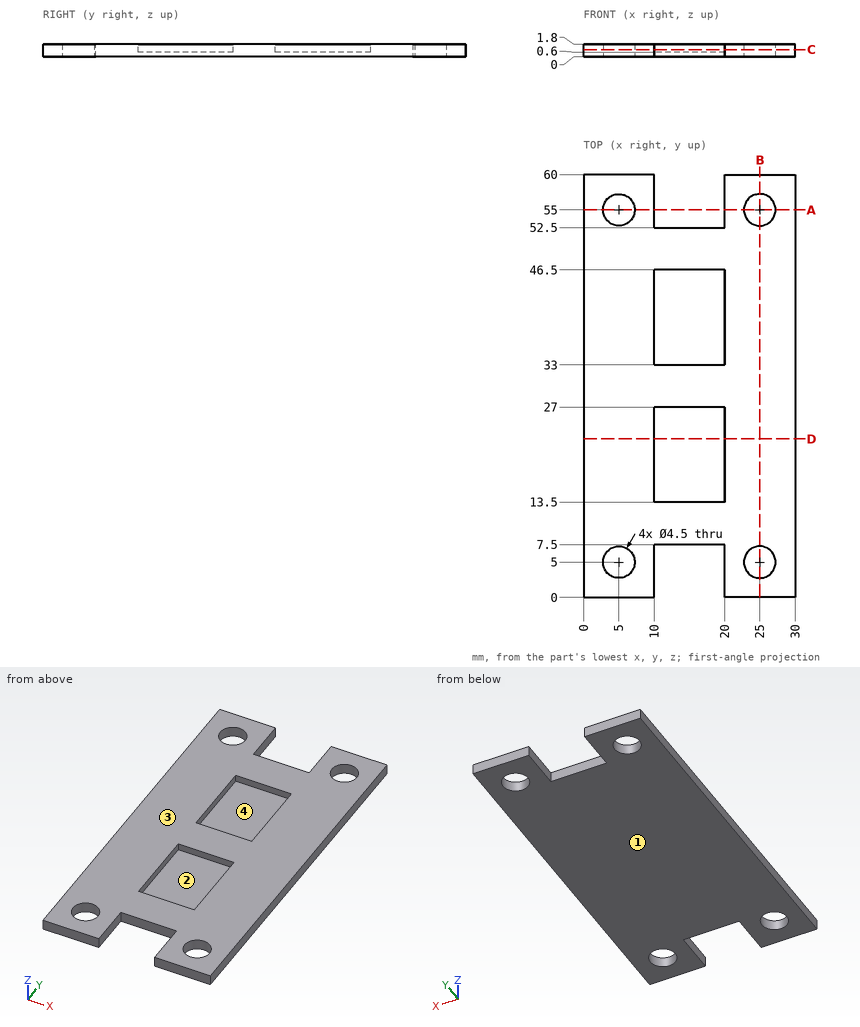
Geometry check sheet. Reference: drawing and pictorial views, mm from the part's lowest x, y, z. A direction names the side the tool comes from. Coordinates: 2 decimals unless noted, no trailing zeros. Order: outer loops, then holes, each group sorted by start corner. A loop starts at its lowest first (then second) coordinate and runs counter-clockwise, first axis right, second up. Notation, with made-up numbers: M 68,29 L 81,29 A28 cw 81,68 Z; hole C -30.75,46.5 d3. An arc over 180 degrees is marked long. Write each question's results on one line, items separated by ' | '. Start each with the question number.
1. Access from +Z, -Z, +X, -X, +Y, -Y to the whole of each face (thin tool, end or side, straight path). Record for the marked faces 3 and 4.
2. Material ranges on probe 1 along Y at (x, z) = (5, 1.4); probe 2 along Y at (x, z) = (17, 1); probe 3 along X at (y, z) = (14, 1.6), recorded low to high.
3. Go/stop test with flat-tipped pins: P1, Ø0.6, axis at y = 17, z = 1.5, coming from the -X side; P2, Ø1, axis at x = 15.5, z = 1, coming from the +Y side; P3, Ø0.5, axis at x = 13, z = 1, coming from the -Y side; P4, Ø3.5, axis at x = 25, y = 5, coming from the +Z side. Record where each tip stops, or that it passes through.
4. Mould release check, pull along X, two halves, no side actions. Record for the marked faces 1 and 2: +X half, -X half, draft (parallel to the pull), parting line (faces both ways), or undercut.
5. Cross-section at C-C on z = 1. Record the cut outline in (x, y).
6. Cross-section at D-D on y = 22.5. Record the cut outline in (x, z), and give its area (3 significant figures).
7. Cross-section at B-B on x = 25. Record the cut outline in (y, z).
8. Cross-section at A-A on y = 55. Record the cut outline in (x, z), and give its area (3 significant figures).
Checks:
1) face 3: +Z, +X, -X, +Y, -Y | face 4: +Z
2) probe 1: y = 0 to 2.75, 7.25 to 52.75, 57.25 to 60 | probe 2: y = 7.5 to 13.5, 27 to 33, 46.5 to 52.5 | probe 3: x = 0 to 10, 20 to 30
3) P1: stops at x = 0 | P2: stops at y = 52.5 | P3: stops at y = 7.5 | P4: passes through
4) face 1: draft | face 2: undercut
5) outline: M 0,0 L 10,0 L 10,7.5 L 20,7.5 L 20,0 L 30,0 L 30,60 L 20,60 L 20,52.5 L 10,52.5 L 10,60 L 0,60 Z; hole C 5,5 d4.5; hole C 5,55 d4.5; hole M 10,13.5 L 20,13.5 L 20,27 L 10,27 Z; hole M 10,33 L 20,33 L 20,46.5 L 10,46.5 Z; hole C 25,5 d4.5; hole C 25,55 d4.5
6) outline: M 0,0 L 30,0 L 30,1.8 L 20,1.8 L 20,0.6 L 10,0.6 L 10,1.8 L 0,1.8 Z | area: 42.0 mm²
7) outline: M 0,0 L 2.75,0 L 2.75,1.8 L 0,1.8 Z; M 7.25,0 L 52.75,0 L 52.75,1.8 L 7.25,1.8 Z; M 57.25,0 L 60,0 L 60,1.8 L 57.25,1.8 Z
8) outline: M 0,0 L 2.75,0 L 2.75,1.8 L 0,1.8 Z; M 7.25,0 L 10,0 L 10,1.8 L 7.25,1.8 Z; M 20,0 L 22.75,0 L 22.75,1.8 L 20,1.8 Z; M 27.25,0 L 30,0 L 30,1.8 L 27.25,1.8 Z | area: 19.8 mm²
